Verification items for the finished model (mm, model axes). A direction names the side the tool comes from. Coordinates: 2 decimals unless noted, no trailing zeros. Order: outer loops, then holes, each group sorted by start corner. A loop starts at its lowest first (then second) coordinate and runs counter-clockwise, first axis right, second up. Notation, with made-up numbers: (-39.75, 41) -> (15.25, 41) arc R31 cw to (15.25, 66) -> close; hole circle Ø7 at (-33, 49.25). An arc over 180 degrees is marked (long way). Answer as CSV lines item,"result".
```python
from build123d import *

# Parameters (mm, degrees)
EXTRUDE_1_DEPTH = 20
FILLET_1_R      = 5


with BuildPart() as part:
    # 草圖1 → 填料-伸長1 (new body)
    with BuildSketch(Plane.XY):
        Polygon((5, 10), (15, 5), (30, 5), (30, 0), (0, 0), (0, 20), (5, 20), align=None)
    extrude(amount=EXTRUDE_1_DEPTH)

    # 圓角1
    fillet_1_edges = [part.edges().sort_by_distance(p)[0] for p in [
        (2.5, 20, 20),
        (30, 2.5, 20),
        (2.5, 20, 0),
        (30, 2.5, 0),
    ]]
    fillet(fillet_1_edges, radius=FILLET_1_R)


solid = part.part
```
Item 1: Section check B-B, the plane x = 2.75. Record the boundary of the cut face in (y, z), plus the area to 3 significant figures.
Answer list:
outline,"(0, 0) -> (15, 0) arc R5 ccw to (20, 5) -> (20, 15) arc R5 ccw to (15, 20) -> (0, 20) -> close"
area,"389 mm2"
Item 2: Depth check by flat-ended pin: pin 1 Ø6 at (x, z) = (11, 15) entering from +Y; pin 2 Ø8 at (y, z) = (13.5, 7.5) entering from +X. Enter the tip coordinate at first touch or a pass-through.
Answer list:
pin 1,"y = 8.5"
pin 2,"x = 6"
Item 3: Thickness scan on line 1 (X direction, y = 13.25, z = 17); line 2 (Y direction, x = 11, z = 4). Record the ranges inside material, lowest first.
Answer list:
line 1,"0 to 5"
line 2,"0 to 7"
Item 4: Section check D-D, the plane z = 17. Record the boundary of the cut face in (x, y), plus the area to 3 significant figures.
Answer list:
outline,"(0, 0) -> (29.58, 0) -> (29.58, 5) -> (15, 5) -> (5, 10) -> (5, 19.58) -> (0, 19.58) -> close"
area,"246 mm2"
Item 5: Section check C-C, the plane y = 7.5. Record the boundary of the cut face in (x, z).
Answer list:
outline,"(0, 0) -> (10, 0) -> (10, 20) -> (0, 20) -> close"
Item 6: Section check A-A, the plane z = 12.75. Record the boundary of the cut face in (x, y).
Answer list:
outline,"(0, 0) -> (30, 0) -> (30, 5) -> (15, 5) -> (5, 10) -> (5, 20) -> (0, 20) -> close"
Item 7: Tool access check on faces 1 (the cylindrical face through (3, 19, 2)), 2 (the flat face through (22, 5, 10)). Record the directions out of +Z, -Z, +X, -X, +Y, -Y that give a thin tool (end or side, any length) a straight path to the whole face; none if there is none.
Answer list:
face 1,"-Z, +X, -X, +Y"
face 2,"+Z, -Z, +X, +Y"
